Answer from the drawing. Dimensions are ordinates in mm from the lowest x, y and z of the part. Coordinates: 2 decimals unless noted, no trailing zeros. Write each loop counter-clockwise with the first axis right and the second up, starting at its lowest first coordinate (ties: lowest second). Pieces come first, ordered by that corner, then holes.
(1) Find the intervals of material crossed by probe 1 along X at (y, z) = (0.8, 4); probe 2 along Z at (x, y) = (5, 0.8); probe 3 along X at (y, z) = (0.1, 3.25), in increasing order.
(2) Section C-C on z = 6.5 is taken. Write down the section's boundary in (x, y), then the cut area to 3 significant figures.
(3) Section D-D on z = 5.25 is taken. Write down the section's boundary in (x, y).
(4) Section B-B on z = 3 is taken. Write down the section's boundary in (x, y).
(5) Section A-A on y = 1.1 is taken. Write down the section's boundary in (x, z), then the cut area to 3 significant figures.
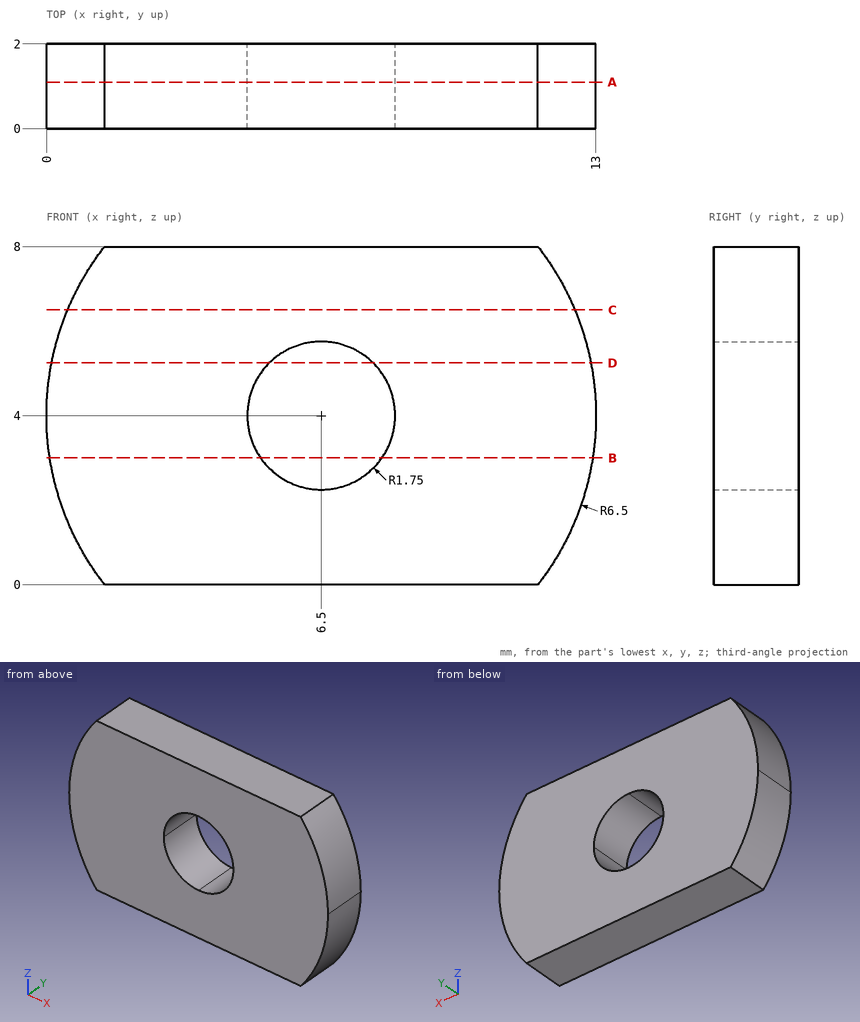
Response:
1. probe 1: x = 0 to 4.75, 8.25 to 13
1. probe 2: z = 0 to 3.1, 4.9 to 8
1. probe 3: x = 0.04 to 4.92, 8.08 to 12.96
2. outline: (0.5, 0) - (12.5, 0) - (12.5, 2) - (0.5, 2) - close
2. area: 24.0 mm2
3. outline: (0.12, 0) - (5.28, 0) - (5.28, 2) - (0.12, 2) - close; (7.72, 0) - (12.88, 0) - (12.88, 2) - (7.72, 2) - close
4. outline: (0.08, 0) - (5.06, 0) - (5.06, 2) - (0.08, 2) - close; (7.94, 0) - (12.92, 0) - (12.92, 2) - (7.94, 2) - close
5. outline: (1.38, 0) - (11.62, 0) arc R6.5 ccw to (11.62, 8) - (1.38, 8) arc R6.5 ccw to start; hole circle Ø3.5 at (6.5, 4)
5. area: 87.4 mm2
